For this review, take the finished solid that the model builds, in its own axes (mm). A direction names the side the tool comes from. Coordinates: 2 decimals unless noted, no trailing zeros. Loops run counter-clockwise (first coordinate to the right, second up) from the corner with the lowest first, then second, coordinate; pieces in that order, holes last. Notation, with made-up numbers: (-7, 83) - (15, 83) arc R4 cw to (15, 90) - close; hole circle Ø4 at (7, 57). An arc over 180 degrees is marked (long way). Use one line per item in the form item = value. Start each with the question number.
1. Add section A-A on y = 61.5. Give the boundary of the cut face in (x, z) (3 decimals).
2. Draft analysis for pull direction X (two halves, no side actions). For faces 1 (the face through (34.724, 53, 14)), 2 (the face through (-55.526, 55, 17)), 3 (the face through (30.028, 68.818, 0.724)), state which applies: +X half, -X half, draft (parallel to the pull), parting line (faces both ways), or undercut.
3. Add section D-D on y = 50.5. Give the boundary of the cut face in (x, z) (3 decimals), and give its area (3 significant figures).
4. Add section C-C on z = 5.25. Give the boundary of the cut face in (x, y).
5. Machinability: for faces 4 (the face through (-16, 55, 6.35)), 5 (the face through (32.382, 66.243, 20.305)), 6 (the face through (-26, 63.232, 4)), 7 (the face through (-26, 42, 25.4)), 8 (the face through (-64, 44.182, 16)), which of the approach directions +Z, -Z, +X, -X, +Y, -Y give a long, thin tool a straight path to every point of the face, cutting with its end or side? Answer none if there is none.
6. To check wall thickness, follow probe 1 along X at (y, z) = (57, 20); probe 2 along X at (y, z) = (48, 19.75); probe 3 along Z at (x, y) = (8, 63). State the ranges of each line that lie inside material, in increasing order.
7. For pin 1 Ø12 at (x, y) = (-10, 61) entering from +Z; pin 2 Ø5.5 at (x, z) = (-64.5, 17) entering from +Y; pin 3 Ø1.5 at (x, z) = (-15.5, 12.5) entering from +Y, all flat-tipped, find the tip position at first contact; note any pin that passes through.
8. Add section B-B on x = -10.5. Give the boundary of the cut face in (y, z), and give its area (3 significant figures).
```python
from build123d import *

# Parameters (mm, degrees)
SKETCH1_W                                = 101.6
SKETCH1_H                                = 25.4
BOSS_EXTRUDE1_DEPTH                      = 25.4
SKETCH2_W                                = 80.725
SKETCH2_H                                = 19.05
CUT_EXTRUDE1_DEPTH                       = 19.05
SKETCH3_W                                = 19.05
SKETCH3_H                                = 19.05
CUT_EXTRUDE2_DEPTH                       = 5
SKETCH4_W                                = 9.525
SKETCH4_H                                = 25.4
BOSS_EXTRUDE2_DEPTH                      = 3.175
SKETCH8_W                                = 9.525
SKETCH8_H                                = 28.575
BOSS_EXTRUDE3_DEPTH                      = 6.35
CBORE_FOR_1_4_HEX_HEAD_BOLT1_D           = 7.14248
CBORE_FOR_1_4_HEX_HEAD_BOLT1_DEPTH       = 9.906
CBORE_FOR_1_4_HEX_HEAD_BOLT1_CBORE_D     = 19.05
CBORE_FOR_1_4_HEX_HEAD_BOLT1_CBORE_DEPTH = 4.7752
CBORE_FOR_1_4_HEX_HEAD_BOLT1_TIP         = 2.145817477
FILLET1_R                                = 2.54


with BuildPart() as part:
    # Sketch1 → Boss-Extrude1 (new body)
    with BuildSketch(Plane.XY):
        with Locations((-16.075949367, 50.532067511)):
            Rectangle(SKETCH1_W, SKETCH1_H)
    extrude(amount=BOSS_EXTRUDE1_DEPTH)

    # Sketch2 → Cut-Extrude1 (cut)
    with BuildSketch(Plane(origin=(0, 63.232067511, 0), x_dir=(1, 0, 0), z_dir=(0, 1, 0))):
        with Locations((-15.163449367, -15.875)):
            Rectangle(SKETCH2_W, SKETCH2_H)
    extrude(amount=-CUT_EXTRUDE1_DEPTH, mode=Mode.SUBTRACT)

    # Sketch3 → Cut-Extrude2 (cut)
    with BuildSketch(Plane.ZY.offset(66.875949367)):
        with Locations((15.875, 53.707067511)):
            Rectangle(SKETCH3_W, SKETCH3_H)
    extrude(amount=-CUT_EXTRUDE2_DEPTH, mode=Mode.SUBTRACT)

    # Sketch4 → Boss-Extrude2 (add)
    with BuildSketch(Plane.XY.offset(25.4)):
        with Locations((29.961550633, 50.532067511)):
            Rectangle(SKETCH4_W, SKETCH4_H)
    extrude(amount=BOSS_EXTRUDE2_DEPTH)

    # Sketch8 → Boss-Extrude3 (add)
    with BuildSketch(Plane(origin=(0, 63.232067511, 0), x_dir=(1, 0, 0), z_dir=(0, 1, 0))):
        with Locations((29.961550633, -14.2875)):
            Rectangle(SKETCH8_W, SKETCH8_H)
    extrude(amount=BOSS_EXTRUDE3_DEPTH)

    # CBORE for 1/4 Hex Head Bolt1
    with Locations(Plane.ZY.offset(-25.199050633)):
        with Locations((22.225, 63.232067511)):
            CounterBoreHole(CBORE_FOR_1_4_HEX_HEAD_BOLT1_D / 2, CBORE_FOR_1_4_HEX_HEAD_BOLT1_CBORE_D / 2, CBORE_FOR_1_4_HEX_HEAD_BOLT1_CBORE_DEPTH, depth=CBORE_FOR_1_4_HEX_HEAD_BOLT1_DEPTH)
            with Locations((0, 0, -(CBORE_FOR_1_4_HEX_HEAD_BOLT1_DEPTH + CBORE_FOR_1_4_HEX_HEAD_BOLT1_TIP / 2))):  # 118° drill point
                Cone(0, CBORE_FOR_1_4_HEX_HEAD_BOLT1_D / 2, CBORE_FOR_1_4_HEX_HEAD_BOLT1_TIP, mode=Mode.SUBTRACT)

    # Fillet1
    fillet1_edges = [part.edges().sort_by_distance(p)[0] for p in [
        (-55.525949367, 44.182067511, 15.875),
        (-15.163449367, 44.182067511, 6.35),
        (-55.525949367, 53.707067511, 6.35),
        (25.199050633, 44.182067511, 15.875),
        (25.199050633, 53.707067511, 6.35),
        (25.199050633, 41.007067511, 25.4),
        (25.199050633, 63.232067511, 3.175),
        (29.961550633, 69.582067511, 0),
    ]]
    fillet(fillet1_edges, radius=FILLET1_R)


solid = part.part
```
Conclusion:
q1.outline = (-66.876, 0) - (34.724, 0) - (34.724, 19.102) - (29.974, 19.102) - (29.974, 12.859) - (25.199, 12.859) - (25.199, 8.89) arc R2.54 cw to (22.659, 6.35) - (-52.986, 6.35) arc R2.54 cw to (-55.526, 8.89) - (-55.526, 25.4) - (-61.876, 25.4) - (-61.876, 6.35) - (-66.876, 6.35) - close; (29.974, 25.348) - (34.724, 25.348) - (34.724, 28.575) - (29.974, 28.575) - close
q2.face_1 = +X half
q2.face_2 = undercut
q2.face_3 = draft
q3.outline = (-66.876, 0) - (34.724, 0) - (34.724, 28.575) - (25.199, 28.575) - (25.199, 8.89) arc R2.54 cw to (22.659, 6.35) - (-52.986, 6.35) arc R2.54 cw to (-55.526, 8.89) - (-55.526, 25.4) - (-61.876, 25.4) - (-61.876, 6.35) - (-66.876, 6.35) - close
q3.area = 981 mm^2
q4.outline = (-66.88, 37.83) - (34.72, 37.83) - (34.72, 69.58) - (25.2, 69.58) - (25.2, 65.77) arc R2.54 cw to (22.66, 63.23) - (-66.88, 63.23) - close
q5.face_4 = +Z, +Y
q5.face_5 = +X
q5.face_6 = +Z, -Z, -X, +Y
q5.face_7 = +Z, -X, +Y, -Y
q5.face_8 = +Z, -X, +Y
q6.probe_1 = -61.88 to -55.53, 29.97 to 34.72
q6.probe_2 = -61.88 to -55.53, 25.2 to 34.72
q6.probe_3 = 0 to 6.35
q7.pin_1 = 6.35
q7.pin_2 = 63.23
q7.pin_3 = 44.18
q8.outline = (37.83, 0) - (63.23, 0) - (63.23, 6.35) - (46.72, 6.35) arc R2.54 cw to (44.18, 8.89) - (44.18, 25.4) - (37.83, 25.4) - close
q8.area = 284 mm^2
